Can you work these out from the model? Positions are in its coordinate system, mm. Face numbers are marked on the shaded views. Coordinates: 2 decimals unless noted, no trailing zeros. Order: outer loops, then holes, each group sorted by start corner. A loop starts at its lowest first (then second) coordinate and runs counter-clockwise, first axis right, second up. Notation, with made-up numbers: (71.25, -14.5) - (75.25, -14.5) arc R23 cw to (75.25, 15.5) - close; hole circle Ø10 at (83, -36.5). An arc over 180 degrees is marked (long way). Use a Markdown table: item, result. Add a question column.
(1) If I drill on L1, parallel to Y at x = 0.05, z = -4; L2, parallel to Y at x = 0, z = 0; L3, parallel to Y at x = -0.1, z = 1.75, over which ranges is the centre line in solid material (lowest first)? Write a range as [from, to].
(2) I want a section at D-D (y = 0). List the corners of the cut face in (x, z) for me, and give its area (3 significant figures).
(3) We'd pull the mould along X, two halves only. Please class the marked faces 1 and 2: pulls with the +X half, pulls with the -X half, needs draft (parallel to the pull), parting line crosses it, or undercut.
(4) I want a section at A-A (z = 0). List the corners of the cut face in (x, y) for me, and give its area (3 significant figures).
(5) I want a section at C-C (z = -1.5). List the corners of the cut face in (x, y) for me.
(6) I want a section at B-B (x = -0.05). List the corners of the cut face in (y, z) for me, and give its area (3 significant figures).
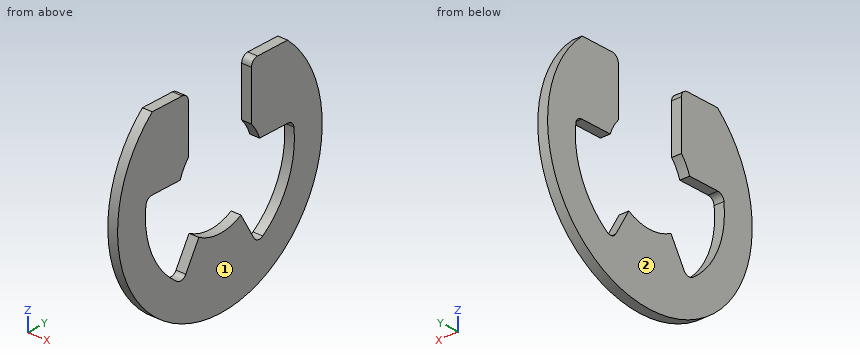
```python
from build123d import *

# Parameters (mm, degrees)
EXTRUDE1_DEPTH = 0.3175
FILLET1_R      = 0.4445


with BuildPart() as part:
    # Sketch1 → Extrude1 (new body, symmetric)
    with BuildSketch(Plane(origin=(0, 0, 0), x_dir=(0, 0, -1), z_dir=(1, 0, 0))):
        with BuildLine():
            Line((-2.03286302, 2.30505), (-5.6007, 2.30505))
            Line((-5.6007, 2.30505), (-5.6007, 4.939353123))
            ThreePointArc((-5.6007, 4.939353123), (7.4676, 0), (-5.6007, -4.939353123))
            Line((-5.6007, -4.939353123), (-5.6007, -2.30505))
            Line((-5.6007, -2.30505), (-2.03286302, -2.30505))
            ThreePointArc((-2.03286302, -2.30505), (-1.557113921, -2.649751648), (-1.024466667, -2.897629308))
            Line((-1.024466667, -2.897629308), (-1.024466667, -5.343190414))
            ThreePointArc((-1.024466667, -5.343190414), (2.262460607, -4.947776041), (4.711625177, -2.720258065))
            Line((4.711625177, -2.720258065), (2.661642476, -1.5367))
            ThreePointArc((2.661642476, -1.5367), (3.0734, 0), (2.661642476, 1.5367))
            Line((2.661642476, 1.5367), (4.711625177, 2.720258065))
            ThreePointArc((4.711625177, 2.720258065), (2.262460607, 4.947776041), (-1.024466667, 5.343190414))
            Line((-1.024466667, 5.343190414), (-1.024466667, 2.897629308))
            ThreePointArc((-1.024466667, 2.897629308), (-1.557113921, 2.649751648), (-2.03286302, 2.30505))
        make_face()
    extrude(amount=EXTRUDE1_DEPTH, both=True)

    # Fillet1
    fillet1_edges = [part.edges().sort_by_distance(p)[0] for p in [
        (0, -2.30505, 5.6007),
        (0, -5.343190414, 1.024466667),
        (0, -2.720258065, -4.711625177),
        (0, 2.720258065, -4.711625177),
        (0, 5.343190414, 1.024466667),
        (0, 2.30505, 5.6007),
    ]]
    fillet(fillet1_edges, radius=FILLET1_R)


solid = part.part
```
Answers follow:
| question | item | result |
|---|---|---|
| 1 | L1 | y = [-6.31, -3.69], [-2.31, 2.31], [3.69, 6.31] |
| 1 | L2 | y = [-7.47, -5.44], [5.44, 7.47] |
| 1 | L3 | y = [-7.26, -2.53], [2.53, 7.26] |
| 2 | outline | (-0.32, -7.47) - (0.32, -7.47) - (0.32, -3.07) - (-0.32, -3.07) - close |
| 2 | area | 2.79 mm² |
| 3 | face 1 | pulls with the +X half |
| 3 | face 2 | pulls with the -X half |
| 4 | outline | (-0.32, -7.47) - (0.32, -7.47) - (0.32, -5.44) - (-0.32, -5.44) - close; (-0.32, 5.44) - (0.32, 5.44) - (0.32, 7.47) - (-0.32, 7.47) - close |
| 4 | area | 2.57 mm² |
| 5 | outline | (-0.32, -7.32) - (0.32, -7.32) - (0.32, -5.23) - (-0.32, -5.23) - close; (-0.32, 5.23) - (0.32, 5.23) - (0.32, 7.32) - (-0.32, 7.32) - close |
| 6 | outline | (-5.4, 0.63) arc R0.44 cw to (-4.96, 1.02) - (-2.9, 1.02) arc R3.07 cw to (-2.31, 2.03) - (-2.31, 5.16) arc R0.44 ccw to (-2.75, 5.6) - (-4.94, 5.6) arc R7.47 ccw (long way) to (4.94, 5.6) - (2.75, 5.6) arc R0.44 ccw to (2.31, 5.16) - (2.31, 2.03) arc R3.07 cw to (2.9, 1.02) - (4.96, 1.02) arc R0.44 cw to (5.4, 0.63) arc R5.44 cw to (3.13, -4.45) arc R0.44 cw to (2.49, -4.31) - (1.54, -2.66) arc R3.07 cw to (-1.54, -2.66) - (-2.49, -4.31) arc R0.44 cw to (-3.13, -4.45) arc R5.44 cw to start |
| 6 | area | 93.8 mm² |
